```python
from build123d import *

# Parameters (mm, degrees)
F1_DEPTH  = 4
F2_DEPTH  = 8
F4_DEPTH  = 59.8075599705
F6_DEPTH  = 59.8075599705
F8_DEPTH  = 59.8075599705
F10_DEPTH = 59.8075599705
F11_F1_R  = 4
F11_F2_R  = 4
F11_F3_R  = 4
F11_F4_R  = 4
F11_F5_R  = 4
F11_F6_R  = 4
F11_F7_R  = 4
F11_F8_R  = 4
F14_DEPTH = 50.75
F15_R     = 7.5


with BuildPart() as f1:
    # F0 (on Right) → F1 (new body)
    with BuildSketch(Plane.YZ):
        Polygon((34.4781084829, 146.4990389768), (30.4781084829, 146.4990389768), (30.4781084829, 22.8514976037), (34.4781084829, 23.1312048515), (34.4781084829, 24.8072521052), (34.4781084829, 40.989404104), (34.4781084829, 85.147008687), (34.4781084829, 101.3291606859), align=None)
        Polygon((109.2856684534, 146.4990389768), (34.4781084829, 146.4990389768), (34.4781084829, 101.3291606859), (94.2856684534, 97.147008687), (94.2856684534, 85.147008687), (34.4781084829, 85.147008687), (34.4781084829, 40.989404104), (94.2856684534, 36.8072521052), (94.2856684534, 24.8072521052), (34.4781084829, 24.8072521052), (34.4781084829, 23.1312048515), (30.4781084829, 22.8514976037), (30.4781084829, 5.3087643873), (109.2856684534, 10.8195258131), (109.2856684534, 54.9771303961), (49.4781084829, 54.9771303961), (49.4781084829, 66.9771303961), (109.2856684534, 71.159282395), (109.2856684534, 115.3168869779), (49.4781084829, 115.3168869779), (49.4781084829, 127.3168869779), (109.2856684534, 131.4990389768), align=None)
        Polygon((109.2856684534, 115.3168869779), (109.2856684534, 131.4990389768), (49.4781084829, 127.3168869779), (49.4781084829, 115.3168869779), align=None)
        Polygon((94.2856684534, 97.147008687), (34.4781084829, 101.3291606859), (34.4781084829, 85.147008687), (94.2856684534, 85.147008687), align=None)
        Polygon((49.4781084829, 54.9771303961), (109.2856684534, 54.9771303961), (109.2856684534, 71.159282395), (49.4781084829, 66.9771303961), align=None)
        Polygon((34.4781084829, 40.989404104), (34.4781084829, 24.8072521052), (94.2856684534, 24.8072521052), (94.2856684534, 36.8072521052), align=None)
        Polygon((113.2856684534, 146.4990389768), (109.2856684534, 146.4990389768), (109.2856684534, 131.4990389768), (109.2856684534, 115.3168869779), (109.2856684534, 71.159282395), (109.2856684534, 54.9771303961), (109.2856684534, 10.8195258131), (30.4781084829, 5.3087643873), (30.4781084829, 0), (113.2856684534, 0), align=None)
        with BuildLine():
            Line((30.4781084829, 0), (30.4781084829, 5.3087643873))
            Line((30.4781084829, 5.3087643873), (12.9781084829, 4.0850451783))
            Line((12.9781084829, 4.0850451783), (12.0231735531, 4.0182696231))
            ThreePointArc((12.0231735531, 4.0182696231), (6.3850122995, 6.0148472379), (4, 11.5))
            ThreePointArc((4, 11.5), (2, 13.5), (0, 11.5))
            ThreePointArc((0, 11.5), (3.3682720164, 3.3682720164), (11.5, 0))
            Line((11.5, 0), (30.4781084829, 0))
        make_face()
        with BuildLine():
            Line((30.4781084829, 5.3087643873), (30.4781084829, 22.8514976037))
            ThreePointArc((30.4781084829, 22.8514976037), (25.4242595831, 10.0215547294), (12.9781084829, 4.0850451783))
            Line((12.9781084829, 4.0850451783), (30.4781084829, 5.3087643873))
        make_face()
    extrude(amount=-F1_DEPTH)

    # F0 (on Right) → F2 (join)
    with BuildSketch(Plane.YZ):
        Polygon((109.2856684534, 115.3168869779), (109.2856684534, 131.4990389768), (49.4781084829, 127.3168869779), (49.4781084829, 115.3168869779), align=None)
        Polygon((94.2856684534, 97.147008687), (34.4781084829, 101.3291606859), (34.4781084829, 85.147008687), (94.2856684534, 85.147008687), align=None)
        Polygon((49.4781084829, 54.9771303961), (109.2856684534, 54.9771303961), (109.2856684534, 71.159282395), (49.4781084829, 66.9771303961), align=None)
        Polygon((34.4781084829, 40.989404104), (34.4781084829, 24.8072521052), (94.2856684534, 24.8072521052), (94.2856684534, 36.8072521052), align=None)
    extrude(amount=F2_DEPTH)

    # F3 (on face) → F4 (cut, through all)
    with BuildSketch(Plane.XZ.offset(-49.4781084829)):
        Polygon((0, 115.3168869779), (8, 115.3168869779), (8, 127.3168869779), align=None)
    extrude(amount=-F4_DEPTH, mode=Mode.SUBTRACT)

    # F5 (on face) → F6 (cut, through all)
    with BuildSketch(Plane(origin=(0, 94.2856684534, 0), x_dir=(-1, 0, 0), z_dir=(0, 1, 0))):
        Polygon((-8, 85.147008687), (0, 85.147008687), (-8, 97.147008687), align=None)
    extrude(amount=-F6_DEPTH, mode=Mode.SUBTRACT)

    # F7 (on face) → F8 (cut, through all)
    with BuildSketch(Plane.XZ.offset(-49.4781084829)):
        Polygon((8, 66.9771303961), (0, 54.9771303961), (8, 54.9771303961), align=None)
    extrude(amount=-F8_DEPTH, mode=Mode.SUBTRACT)

    # F9 (on face) → F10 (cut, through all)
    with BuildSketch(Plane(origin=(0, 94.2856684534, 0), x_dir=(-1, 0, 0), z_dir=(0, 1, 0))):
        Polygon((0, 24.8072521052), (-8, 36.8072521052), (-8, 24.8072521052), align=None)
    extrude(amount=-F10_DEPTH, mode=Mode.SUBTRACT)

    # F11: fillet of radius 4 on 8 edges, made by hand

    # F11_f1
    f11_f1_edges = [f1.edges().sort_by_distance(p)[0] for p in [
        (4, 94.2856684534, 36.8072521052),
    ]]
    fillet(f11_f1_edges, radius=F11_F1_R)

    # F11_f2
    f11_f2_edges = [f1.edges().sort_by_distance(p)[0] for p in [
        (8, 63.1041505096, 36.8072521052),
    ]]
    fillet(f11_f2_edges, radius=F11_F2_R)

    # F11_f3
    f11_f3_edges = [f1.edges().sort_by_distance(p)[0] for p in [
        (4, 49.4781084829, 66.9771303961),
    ]]
    fillet(f11_f3_edges, radius=F11_F3_R)

    # F11_f4
    f11_f4_edges = [f1.edges().sort_by_distance(p)[0] for p in [
        (8, 80.6596264267, 66.9771303961),
    ]]
    fillet(f11_f4_edges, radius=F11_F4_R)

    # F11_f5
    f11_f5_edges = [f1.edges().sort_by_distance(p)[0] for p in [
        (4, 94.2856684534, 97.147008687),
    ]]
    fillet(f11_f5_edges, radius=F11_F5_R)

    # F11_f6
    f11_f6_edges = [f1.edges().sort_by_distance(p)[0] for p in [
        (8, 63.1041505096, 97.147008687),
    ]]
    fillet(f11_f6_edges, radius=F11_F6_R)

    # F11_f7
    f11_f7_edges = [f1.edges().sort_by_distance(p)[0] for p in [
        (4, 49.4781084829, 127.3168869779),
    ]]
    fillet(f11_f7_edges, radius=F11_F7_R)

    # F11_f8
    f11_f8_edges = [f1.edges().sort_by_distance(p)[0] for p in [
        (8, 80.6596264267, 127.3168869779),
    ]]
    fillet(f11_f8_edges, radius=F11_F8_R)


with BuildPart() as f12_1:
    # F12: instance of F1
    add(f1.part.mirror(Plane(origin=(0, 70.5723781379, 70.1443425212), x_dir=(0, 1, 0), z_dir=(1, 0, 0))))


with BuildPart() as f12_1_1:
    # F13: moved
    add(f12_1.part.moved(Location((50.75, 0, 0))))


with BuildPart() as f1_1:
    add(f1.part)

    add(f12_1_1.part)  # F14 merges F12_1
    # F0 (on Right) → F14 (join, through all)
    with BuildSketch(Plane.YZ):
        Polygon((34.4781084829, 146.4990389768), (30.4781084829, 146.4990389768), (30.4781084829, 22.8514976037), (34.4781084829, 23.1312048515), (34.4781084829, 24.8072521052), (34.4781084829, 40.989404104), (34.4781084829, 85.147008687), (34.4781084829, 101.3291606859), align=None)
        Polygon((113.2856684534, 146.4990389768), (109.2856684534, 146.4990389768), (109.2856684534, 131.4990389768), (109.2856684534, 115.3168869779), (109.2856684534, 71.159282395), (109.2856684534, 54.9771303961), (109.2856684534, 10.8195258131), (30.4781084829, 5.3087643873), (30.4781084829, 0), (113.2856684534, 0), align=None)
        with BuildLine():
            Line((30.4781084829, 0), (30.4781084829, 5.3087643873))
            Line((30.4781084829, 5.3087643873), (12.9781084829, 4.0850451783))
            Line((12.9781084829, 4.0850451783), (12.0231735531, 4.0182696231))
            ThreePointArc((12.0231735531, 4.0182696231), (6.3850122995, 6.0148472379), (4, 11.5))
            ThreePointArc((4, 11.5), (2, 13.5), (0, 11.5))
            ThreePointArc((0, 11.5), (3.3682720164, 3.3682720164), (11.5, 0))
            Line((11.5, 0), (30.4781084829, 0))
        make_face()
    extrude(amount=F14_DEPTH)

    # F15
    f15_edges = [f1_1.edges().sort_by_distance(p)[0] for p in [
        (4, 109.285668, 131.499039),
        (4, 109.285668, 71.159282),
        (46.75, 109.285668, 71.159282),
        (46.75, 109.285668, 131.499039),
        (4, 34.478108, 40.989404),
        (4, 34.478108, 101.329161),
        (46.75, 34.478108, 40.989404),
        (46.75, 34.478108, 101.329161),
        (25.375, 109.285668, 10.819526),
    ]]
    fillet(f15_edges, radius=F15_R)


solid = f1_1.part
```
The model under review builds one solid part; all positions refer to its coordinate system, in mm. A direction names the side the tool comes from. Round coordinates to 2 decimals unless told otherwise and drop trailing zeros. Loops run counter-clockwise (first coordinate to the right, second up) from the corner with the lowest first, then second, coordinate; pieces in that order, holes last. Notation, with made-up numbers: M 76,-6 L 81,-6 A26 ccw 81,9 Z; hole C 70,-39 d9. An arc over 180 degrees is marked long. Put each result on its own line as item: value.
Q1. Mouldability with a two-part tool opening along Z and no side actions: class faces 4 (the flat face through (42.75, 96, 70)), 5 (the flat face through (46.81, 66.35, 99.1)), 6 (the flat face through (51, 75, 146.499)) as released by +Z, released by -Z, zero draft, split by the parting line, or undercut.
Result set:
face 4: zero draft
face 5: undercut
face 6: released by +Z
Q2. Consider section A-A, the plane x = 24.5. Give the boundary of the cut face in (y, z), then the cut area to 3 significant figures.
Result set:
outline: M 0,11.5 A11.5 ccw 11.5,0 L 113.29,0 L 113.29,146.5 L 109.29,146.5 L 109.29,17.81 A7.5 cw 102.31,10.33 L 12.02,4.02 A7.5 cw 4,11.5 A2 ccw Z; M 30.48,22.85 L 34.48,23.13 L 34.48,146.5 L 30.48,146.5 Z
area: 1,880 mm²
Q3. To check wall thickness, follow L1, parallel to Y at x = 13, z = 37; L2, parallel to X at y = 105, z = 130.5; L3, parallel to X at y = 97.5, z = 27.5. State the ranges of each line that lie inside material, in increasing order.
Result set:
L1: y = 30.48 to 34.48, 109.29 to 113.29
L2: x = -4 to 8, 42.75 to 54.75
L3: x = -4 to 0, 50.75 to 54.75
Q4. Consider section B-B, the plane z = 80. Give the boundary of the cut face in (x, y), then the cut area to 3 significant figures.
Result set:
outline: M -4,30.48 L 54.75,30.48 L 54.75,113.29 L -4,113.29 Z; hole M 0,34.48 L 50.75,34.48 L 50.75,109.29 L 0,109.29 Z
area: 1,070 mm²
Q5. Machinability: for faces 1 (the cylindrical face through (46.752, 50.582, 126.345)), 2 (the flat face through (47.137, 64.801, 30.226)), 3 (the flat face through (54.75, 68, 74)), which of the approach directions +Z, -Z, +X, -X, +Y, -Y give a long, thin tool a straight path to every point of the face, cutting with its end or side? Answer none if there is none.
Result set:
face 1: +Z
face 2: none
face 3: +Z, -Z, +X, +Y, -Y
Q6. Consider section C-C, the plane y = 25. Give the boundary of the cut face in (x, z).
Result set:
outline: M -4,0 L 54.75,0 L 54.75,9.58 L 50.75,9.58 L 50.75,4.93 L 0,4.93 L 0,9.58 L -4,9.58 Z
Q7. Consider section D-D, the plane z = 21. Give the boundary of the cut face in (x, y).
Result set:
outline: M -4,30.39 L 0,30.39 L 0,109.29 L 50.75,109.29 L 50.75,30.39 L 54.75,30.39 L 54.75,113.29 L -4,113.29 Z
Q8. For pin 1 (4.5 mm diameter, centred on x = 49, z = 121, fed in from -Y); pin 2 (10 mm diameter, centred on x = 41, z = 15.5, fed in from -Y), all flat-tipped, find the tip position at first contact; note any pin that passes through.
Result set:
pin 1: stops at y = 30.48
pin 2: stops at y = 0
